Read the model definition and answer for the solid it produces. Units are mm, in the model's axes. Coordinates: 2 decimals unless noted, no trailing zeros. Write each loop counter-clockwise with the first axis right and the second up, starting at its lowest first coordinate (ties: lowest second). Pieces come first, ordered by that corner, then holes. Notation, with made-up numbers: (72.25, 10.5) - (87.25, 10.5) arc R8 ccw to (87.25, 16.5) - close; hole circle Ø9 at (68, 35.25). An arc over 180 degrees is marked (long way). Return JSON: item names as keys, results as strings.
```python
from build123d import *

# Parameters (mm, degrees)
SKETCH1_W           = 10
SKETCH1_H           = 5
SKETCH1_W_2         = 5
SKETCH1_H_2         = 15
BOSS_EXTRUDE1_DEPTH = 5
FILLET2_R           = 20


with BuildPart() as part:
    # Sketch1 → Boss-Extrude1 (new body)
    with BuildSketch(Plane(origin=(0, 0, 0), x_dir=(1, 0, 0), z_dir=(0, 1, 0))):
        Polygon((-30.064538889, 111.027213551), (-25.064538889, 111.027213551), (-25.064538889, 62.527213551), (-5.064538889, 62.527213551), (-5.064538889, 141.027213551), (-30.064538889, 141.027213551), align=None)
        with Locations((-15.064538889, 70.027213551)):
            Rectangle(SKETCH1_W, SKETCH1_H, mode=Mode.SUBTRACT)
        with Locations((-25.064538889, 126.027213551)):
            Rectangle(SKETCH1_W_2, SKETCH1_H_2, mode=Mode.SUBTRACT)
    extrude(amount=BOSS_EXTRUDE1_DEPTH)

    # Fillet2
    fillet2_edges = [part.edges().sort_by_distance(p)[0] for p in [
        (-5.064538889, 2.5, -141.027213551),
    ]]
    fillet(fillet2_edges, radius=FILLET2_R)


solid = part.part
```
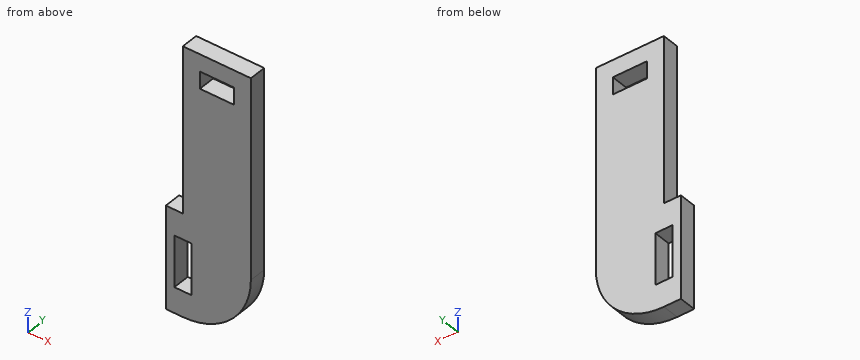
(1) A cutting plane is placed at A-A (x = -25.75). Determine the outline of the cut face in (y, z), and give its area (3 significant figures).
Answer:
{"outline": "(0, -141.03) - (5, -141.03) - (5, -133.53) - (0, -133.53) - close; (0, -118.53) - (5, -118.53) - (5, -111.03) - (0, -111.03) - close", "area": "75.0 mm²"}
(2) A cutting plane is placed at D-D (z = -85.5). Determine the outline of the cut face in (x, y), and give its area (3 significant figures).
Answer:
{"outline": "(-25.06, 0) - (-5.06, 0) - (-5.06, 5) - (-25.06, 5) - close", "area": "100 mm²"}
(3) Straight lines are drawn through the part: line 1 (Z direction, x = -26, y = 3.35); line 2 (X direction, y = 2.35, z = -119.5); line 3 (Z direction, x = -19.25, y = 1.4). For each, find the intervals that lie inside material, in ascending order. Write a range as from..to.
Answer:
{"line 1": "-141.03..-133.53, -118.53..-111.03", "line 2": "-30.06..-27.56, -22.56..-5.06", "line 3": "-140.16..-72.53, -67.53..-62.53"}
(4) Flat-ended cylindrical pins translate along their axes: P1, Ø2.5, axis at x = -27, y = 3.5, coming from the +Z side; P2, Ø1.5, axis at x = -14.5, y = 2.5, coming from the -Z side; P3, Ø1.5, axis at y = 1.5, z = -71, coming from the -X side. Find the tip coordinate at first contact, or state that the pin passes through.
Answer:
{"P1": "z = -111.03", "P2": "z = -138.45", "P3": "x = -25.06"}
(5) A cutting plane is placed at C-C (z = -128.5). Determine the outline of the cut face in (x, y).
Answer:
{"outline": "(-30.06, 0) - (-27.56, 0) - (-27.56, 5) - (-30.06, 5) - close; (-22.56, 0) - (-6.51, 0) - (-6.51, 5) - (-22.56, 5) - close"}
(6) A cutting plane is placed at B-B (y = 0.7). Determine the outline of the cut face in (x, z).
Answer:
{"outline": "(-30.06, -141.03) - (-25.06, -141.03) arc R20 ccw to (-5.06, -121.03) - (-5.06, -62.53) - (-25.06, -62.53) - (-25.06, -111.03) - (-30.06, -111.03) - close; hole (-27.56, -133.53) - (-22.56, -133.53) - (-22.56, -118.53) - (-27.56, -118.53) - close; hole (-20.06, -72.53) - (-10.06, -72.53) - (-10.06, -67.53) - (-20.06, -67.53) - close"}
